Source: CAD feature listing. Evaluate the final solid. Frame: model axes, mm. Face numbers are marked on the shaded views. A direction names the side the tool comes from. Give positions to 0.01 mm unless a question says otherwise; leave off trailing zeros. Return JSON: item names as keys, results as strings.
```python
from build123d import *

# Parameters (mm, degrees)
F3_ANGLE_BACK   = 5
F3_ANGLE        = 10
F5_D            = 5.5
F5_COPIES_COUNT = 3
F8_ANGLE_BACK   = 5
F8_ANGLE        = 10


# Not quite as in the source:
# - a pattern or mirror of a feature is missing from the dataset's text; its kind, count and spacing are read off the source's solid


with BuildPart() as f1:
    # F0 (on Front) → F1 (revolve)
    with BuildSketch(Plane.XZ):
        with BuildLine():
            Line((41.9487010796, 5), (14.25, 5))
            Line((14.25, 5), (14.25, 21))
            Line((14.25, 21), (6.25, 21))
            Line((6.25, 21), (6.25, 0))
            Line((6.25, 0), (50, 0))
            ThreePointArc((50, 0), (49.4855209657, 9.058253519), (47.9487010796, 18))
            Line((47.9487010796, 18), (41.9487010796, 18))
            Line((41.9487010796, 18), (41.9487010796, 5))
        make_face()
    revolve(axis=Axis((0, 0, 8.5228504971), (0, 0, 1)))

    # F2 (on Front) → F3 (revolve)
    with BuildSketch(Plane.XZ, mode=Mode.PRIVATE) as f3_sk:
        Polygon((-14.25, 21), (-41.9487010796, 18), (-41.9487010796, 5), (-14.25, 5), align=None)
    f3 = revolve(f3_sk.sketch.rotate(Axis((0, 0, 5), (0, 0, 1)), -F3_ANGLE_BACK), axis=Axis((0, 0, 5), (0, 0, 1)), revolution_arc=F3_ANGLE)

    # F3_copies: F3 across plane
    add(f3.mirror(Plane(origin=(0, 0, 0), x_dir=(0.5, 0.8660254038, 0), z_dir=(0.8660254038, -0.5, 0))))

    # F5 (through all)
    with Locations(Plane.XY.offset(5)):
        with Locations((30, 0)):
            f5 = Hole(F5_D / 2)

    # F5_copies: F5 ×3 about axis
    f5_copies_axis = Axis((0, 0, 0), (0, 0, 1))
    for i in range(1, F5_COPIES_COUNT):
        add(f5.rotate(f5_copies_axis, i * 360 / F5_COPIES_COUNT), mode=Mode.SUBTRACT)

    # F7 (on face) → F8 (revolve)
    with BuildSketch(Plane(origin=(0, 0, 0), x_dir=(0.5, 0.8660254038, 0), z_dir=(0.8660254038, -0.5, 0)), mode=Mode.PRIVATE) as f8_sk:
        Polygon((14.25, 5), (41.9487010796, 5), (41.9487010796, 18), (14.25, 21), align=None)
    revolve(f8_sk.sketch.rotate(Axis((0, 0, 5), (0, 0, 1)), -F8_ANGLE_BACK), axis=Axis((0, 0, 5), (0, 0, 1)), revolution_arc=F8_ANGLE)


solid = f1.part
```
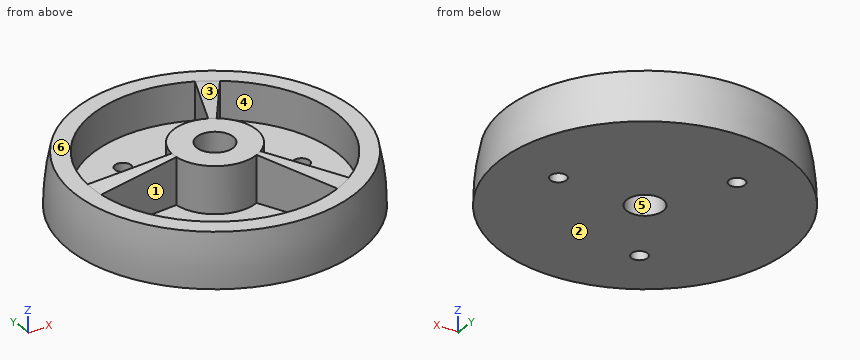
1) Draft query along Y for the marked faces 1, 2, 3 and 4. Return one class per face: released by +Y, released by -Y, zero draft, split by the parting line, or undercut.
Numbers:
{"face 1": "undercut", "face 2": "zero draft", "face 3": "released by +Y", "face 4": "undercut"}
2) Line query: line 1 (X direction, y = -28, z = 7.5); line 2 (X direction, y = -5, z = 14.25); line 3 (X direction, y = -26, z = 13.5). Output: solid intervals per line, ascending. Write a range as [from, to].
Numbers:
{"line 1": "x = [-41, -31.24], [13.06, 19.61], [31.24, 41]", "line 2": "x = [-48.46, -41.65], [-13.34, -3.75], [3.75, 13.34], [41.65, 48.46]", "line 3": "x = [-41.36, -32.92], [12.12, 18.21], [32.92, 41.36]"}
3) Contact query for flat-ended pins moving along their axis: pin 1 Ø3 at (x, z) = (34, 6) entering from +Y; pin 2 Ø7.5 at (x, y) = (0, 0) entering from +Z (3 decimals); pin 3 Ø10 at (x, y) = (31, 10.5) entering from +Z; pin 4 Ø6 at (x, y) = (-36.5, -3) entering from +Z. Output: stop coordinate, or through.
Numbers:
{"pin 1": "stops at y = 37.71", "pin 2": "passes through", "pin 3": "stops at z = 5", "pin 4": "stops at z = 18.9"}
4) Set-up query: the marked faces 5 and 6. Return all of +Z, -Z, +X, -X, +Y, -Y with unobstructed straight access to the full face (end or side cutting, diameter ignored); none if empty.
Numbers:
{"face 5": "+Z, -Z", "face 6": "+Z"}
5) Cut plane A-A, the plane y = 0. Give the number of separate pieces and of enclosed holes in the cut face, then the cut area to 3 significant figures.
Numbers:
{"separate pieces": "3", "enclosed holes": "0", "area": "1,250 mm²"}
